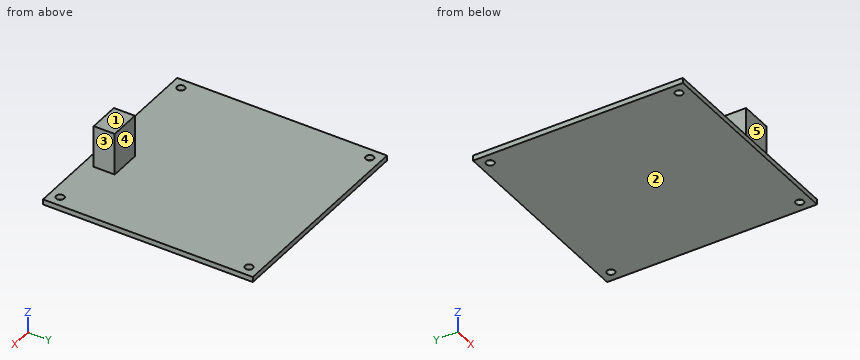
Solid Edge part; units mm, degrees
sketch "Sketch1" plane through (0, 0, 0) normal (0, 0, 1) x (1, 0, 0)
  line L0 (-63.5, -63.5) -> (63.5, -63.5)
  line L1 (63.5, -63.5) -> (63.5, 63.5)
  line L2 (63.5, 63.5) -> (-63.5, 63.5)
  line L3 (-63.5, 63.5) -> (-63.5, -63.5)
  dimension "D1" = 63.5
  dimension "D2" = 63.5
extrude "Protrusion1" add sketch "Sketch1" along normal blind 3.175
hole "Hole_1" at (-57.15, 57.15, 3.175) direction (0, 0, -1) diameter 4.7625 end up to next
hole "Hole1" at (57.15, 57.15, 3.175) direction (0, 0, -1) diameter 4.7625 end up to next
hole "Hole2" at (57.15, -57.15, 3.175) direction (0, 0, -1) diameter 4.7625 end up to next
hole "Hole3" at (-57.15, -57.15, 3.175) direction (0, 0, -1) diameter 4.7625 end up to next
sketch "Sketch2" plane through (0, 0, 3.175) normal (0, 0, 1) x (0, -1, 0)
  line L0 (44.45, 6.35) -> (57.15, 6.35)
  line L1 (57.15, 6.35) -> (57.15, 25.4)
  line L2 (57.15, 25.4) -> (44.45, 25.4)
  line L3 (44.45, 25.4) -> (44.45, 6.35)
  dimension "D1" = 57.15
  dimension "D2" = 44.45
extrude "ExtrudedProtrusion_2" add sketch "Sketch2" along normal blind 25.4
properties material "ABS Plastic, high impact"
Geometry check sheet. Reference: the model listing, model coordinates, mm. Face numbers are marked on the shaded views. A direction names the side the tool comes from. Round coordinates to 2 decimals unless told otherwise and drop trailing zeros. Loops run counter-clockwise (first coordinate to the right, second up) from the corner with the lowest first, then second, coordinate; pieces in that order, holes last.
Item 1: Access from +Z, -Z, +X, -X, +Y, -Y to the whole of each face (thin tool, end or side, straight path). Record for the marked faces 1, 2, 3, 4 and 5.
Item 2: Thickness scan on line 1 (Y direction, x = -57.15, z = 0.75); line 2 (Z direction, x = 20, y = -5.5) (3 decimals). Record the ranges inside material, lowest first.
Item 3: Cross-section at A-A on x = 57.15. Record the boundary of the cut face in (y, z) (3 decimals).
Item 4: Gauge pin test, flat ends, axial feed: pin 1 (12 mm diameter, centred on x = 16, y = 31, fed in from +Z) (3 decimals); pin 2 (6 mm diameter, centred on x = 45, z = 6, fed in from +Y); pin 3 (15 mm diameter, centred on x = 18.5, z = 20.5, fed in from -Y); pin 4 (10 mm diameter, centred on y = -54, z = 20, fed in from +X). Record the tip position at first contact, or that the pin passes through.
Item 5: Cross-section at D-D on z = 25.5. Record the boundary of the cut face in (x, y).
Item 6: Cross-section at C-C on x = 18. Record the boundary of the cut face in (y, z) (3 decimals), then the cut area to 3 significant figures.
Answer sheet:
1. face 1: +Z, +X, -X, +Y, -Y
1. face 2: -Z, +X, -X, +Y, -Y
1. face 3: +Z, +X, +Y, -Y
1. face 4: +Z, +X, -X, +Y
1. face 5: +Z, +X, -X, -Y
2. line 1: y = -63.5 to -59.53, -54.77 to 54.77, 59.53 to 63.5
2. line 2: z = 0 to 3.175
3. outline: (-63.5, 0) - (-59.531, 0) - (-59.531, 3.175) - (-63.5, 3.175) - close; (-54.769, 0) - (54.769, 0) - (54.769, 3.175) - (-54.769, 3.175) - close; (59.531, 0) - (63.5, 0) - (63.5, 3.175) - (59.531, 3.175) - close
4. pin 1: stops at z = 3.175
4. pin 2: stops at y = 63.5
4. pin 3: stops at y = -57.15
4. pin 4: stops at x = 25.4
5. outline: (6.35, -57.15) - (25.4, -57.15) - (25.4, -44.45) - (6.35, -44.45) - close
6. outline: (-63.5, 0) - (63.5, 0) - (63.5, 3.175) - (-44.45, 3.175) - (-44.45, 28.575) - (-57.15, 28.575) - (-57.15, 3.175) - (-63.5, 3.175) - close
6. area: 726 mm2
